Verification items for the finished model (mm, model axes). Round coordinates to 2 decimals unless told otherwise and drop trailing zeros. Write each loop counter-clockwise with the first axis right and the second up, starting at its lowest first coordinate (ties: lowest second). Pieces come first, ordered by that corner, then holes. Notation, with made-up numbers: M 34.25,73.25 L 82.25,73.25 A34 cw 82.25,111.25 Z; hole C 22,54.25 d4. An arc over 180 degrees is marked long. Write each question's results on one line, items separated by ' | '.
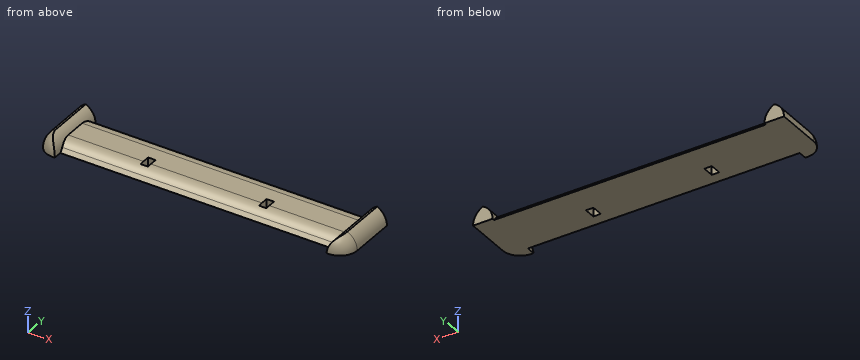
from build123d import *

# Parameters (mm, degrees)
F0_W          = 90
F0_H          = 18.32
F1_DEPTH      = 2.5
F2_W          = 2.16
F2_H          = 3.27
F3_DEPTH      = 25
F4_W          = 5
F4_H          = 18.32
F5_DEPTH      = 2.5
F6_T1_DEPTH   = 43.32
F6_T3_DEPTH   = 39.9706350946
F7_T1_DEPTH   = 39.9706350946
F7_T3_DEPTH   = 43.32
F8_T4_DEPTH   = 105.7168298797
F8_S5_R       = 5.0000000001
F8_T6_DEPTH   = 54
F8_S7_R       = 5.0000000001
F8_T8_DEPTH   = 54
F9_T4_DEPTH   = 105
F9_S5_R       = 5.0000000001
F9_T6_DEPTH   = 54
F9_S7_R       = 5.0000000001
F9_T8_DEPTH   = 54
F10_T4_ANGLE  = 350.8787991533
F10_S5_R      = 5.0000000001
F10_T6_DEPTH  = 9
F10_T10_ANGLE = 350.8787991654
F10_S11_R     = 5.0000000001
F10_T12_DEPTH = 9
F11_T4_DEPTH  = 90.3553390593
F11_S5_R      = 5.0000000001
F11_T6_DEPTH  = 47
F11_S7_R      = 5.0000000001
F11_T8_DEPTH  = 47


# Not quite as in the source:
# - a fillet or chamfer that OpenCascade refuses, or shapes differently, is made with other operations: its cross-section is extruded or revolved along the edge and cut away or added


with BuildPart() as f1:
    # F0 (on Top) → F1 (new body)
    with BuildSketch(Plane.XY):
        with Locations((28.5399998152, 34.3848172414)):
            Rectangle(F0_W, F0_H)
    extrude(amount=F1_DEPTH)

    # F2 (on face) → F3 (cut)
    with BuildSketch(Plane(origin=(0, 0, 0), x_dir=(1, 0, 0), z_dir=(0, 0, -1))):
        with Locations((11.4099998152, -32.7498172414)):
            Rectangle(F2_W, F2_H)
        with Locations((45.6699998152, -32.7498172414)):
            Rectangle(F2_W, F2_H)
    extrude(amount=-F3_DEPTH, mode=Mode.SUBTRACT)

    # F4 (on face) → F5 (join)
    with BuildSketch(Plane.XY.offset(2.5)):
        with Locations((-13.9600001848, 34.3848172414)):
            Rectangle(F4_W, F4_H)
        with Locations((71.0399998152, 34.3848172414)):
            Rectangle(F4_W, F4_H)
    extrude(amount=F5_DEPTH)

    # F6: fillet of radius 5 on 2 edges, made by hand

    # F6_s2 → F6_t1 (cut)
    with BuildSketch(Plane.XZ.offset(-56.0448172414)):
        with BuildLine():
            ThreePointArc((-16.4600001848, 0), (-14.9955340907, 3.5355339059), (-11.4600001848, 5))
            Line((-11.4600001848, 5), (-16.4600001848, 5))
            Line((-16.4600001848, 5), (-16.4600001848, 0))
        make_face()
    extrude(amount=F6_T1_DEPTH, mode=Mode.SUBTRACT)

    # F6_s4 → F6_t3 (cut)
    with BuildSketch(Plane.XZ.offset(-54.3701347887)):
        with BuildLine():
            ThreePointArc((-15.7901272037, 5), (-13.2901272037, 4.3301270189), (-11.4600001848, 2.5))
            Line((-11.4600001848, 2.5), (-11.4600001848, 5))
            Line((-11.4600001848, 5), (-15.7901272037, 5))
        make_face()
    extrude(amount=F6_T3_DEPTH, mode=Mode.SUBTRACT)

    # F7: fillet of radius 5 on 2 edges, made by hand

    # F7_s2 → F7_t1 (cut)
    with BuildSketch(Plane.XZ.offset(-54.3701347887)):
        with BuildLine():
            ThreePointArc((68.5399998152, 2.5), (70.3701268341, 4.3301270189), (72.8701268341, 5))
            Line((72.8701268341, 5), (68.5399998152, 5))
            Line((68.5399998152, 5), (68.5399998152, 2.5))
        make_face()
    extrude(amount=F7_T1_DEPTH, mode=Mode.SUBTRACT)

    # F7_s4 → F7_t3 (cut)
    with BuildSketch(Plane.XZ.offset(-56.0448172414)):
        with BuildLine():
            ThreePointArc((73.5399998152, 0), (72.0755337212, 3.5355339059), (68.5399998152, 5))
            Line((68.5399998152, 5), (73.5399998152, 5))
            Line((73.5399998152, 5), (73.5399998152, 0))
        make_face()
    extrude(amount=F7_T3_DEPTH, mode=Mode.SUBTRACT)

    # F8: chamfer of 5 on 1 edges, made by hand


with BuildPart() as f8_tool2:
    # F8_s3 → F8_t4 (new body)
    with BuildSketch(Plane.YZ.offset(-24.3184151246)):
        Polygon((30.2248172414, 2.5), (25.2248172414, -2.5), (25.2248172414, 2.5), align=None)
    extrude(amount=F8_T4_DEPTH)

    # F8_s5 → F8_t6 (cut, symmetric)
    with BuildSketch(Plane.XZ.offset(-27.7)):
        with Locations((-15.7901272038, -1e-10)):
            Circle(F8_S5_R)
    extrude(amount=F8_T6_DEPTH, both=True, mode=Mode.SUBTRACT)

    # F8_s7 → F8_t8 (cut, symmetric)
    with BuildSketch(Plane.XZ.offset(-27.7)):
        with Locations((72.8701268342, -1e-10)):
            Circle(F8_S7_R)
    extrude(amount=F8_T8_DEPTH, both=True, mode=Mode.SUBTRACT)


with BuildPart() as f1_1:
    add(f1.part)

    # F8_t1: cut F8_tool2
    add(f8_tool2.part, mode=Mode.SUBTRACT)

    # F9: fillet of radius 5 on 1 edges, made by hand


with BuildPart() as f9_tool2:
    # F9_s3 → F9_t4 (new body)
    with BuildSketch(Plane.YZ.offset(81.0399998152)):
        with BuildLine():
            ThreePointArc((43.5448172414, -2.5), (42.0803511473, 1.0355339059), (38.5448172414, 2.5))
            Line((38.5448172414, 2.5), (43.5448172414, 2.5))
            Line((43.5448172414, 2.5), (43.5448172414, -2.5))
        make_face()
    extrude(amount=-F9_T4_DEPTH)

    # F9_s5 → F9_t6 (cut, symmetric)
    with BuildSketch(Plane.XZ.offset(-41)):
        with Locations((72.8701268342, -1e-10)):
            Circle(F9_S5_R)
    extrude(amount=F9_T6_DEPTH, both=True, mode=Mode.SUBTRACT)

    # F9_s7 → F9_t8 (cut, symmetric)
    with BuildSketch(Plane.XZ.offset(-41)):
        with Locations((-15.7901272038, -1e-10)):
            Circle(F9_S7_R)
    extrude(amount=F9_T8_DEPTH, both=True, mode=Mode.SUBTRACT)


with BuildPart() as f1_2:
    add(f1_1.part)

    # F9_t1: cut F9_tool2
    add(f9_tool2.part, mode=Mode.SUBTRACT)

    # F10: fillet of radius 5 on 2 edges, made by hand


with BuildPart() as f10_tool2:
    # F10_s3 → F10_t4 (revolve)
    with BuildSketch(Plane(origin=(-4.0989769567, 0, -5.492965009), x_dir=(0, 1, 0), z_dir=(0.5980609221, 0, 0.8014506432))):
        with BuildLine():
            ThreePointArc((25.2248172414, 9.1846245187), (26.6892833355, 5.6490906128), (30.2248172414, 4.1846245187))
            Line((30.2248172414, 4.1846245187), (25.2248172414, 4.1846245187))
            Line((25.2248172414, 4.1846245187), (25.2248172414, 9.1846245187))
        make_face()
    revolve(axis=Axis((-11.4600001847, 25.2248172414, -1e-10), (0, 1, 0)), revolution_arc=F10_T4_ANGLE)

    # F10_s5 → F10_t6 (intersect, symmetric)
    with BuildSketch(Plane.XZ.offset(-27.7)):
        with Locations((-15.7901272038, -1e-10)):
            Circle(F10_S5_R)
    extrude(amount=F10_T6_DEPTH, both=True, mode=Mode.INTERSECT)


with BuildPart() as f1_3:
    add(f1_2.part)

    # F10_t1: cut F10_tool2
    add(f10_tool2.part, mode=Mode.SUBTRACT)


with BuildPart() as f10_tool8:
    # F10_s9 → F10_t10 (revolve)
    with BuildSketch(Plane(origin=(14.7214175546, 0, -28.147572216), x_dir=(0, 1, 0), z_dir=(0.4634498715, 0, -0.8861231385))):
        with BuildLine():
            ThreePointArc((25.2248172414, 60.7348797497), (26.6892833355, 57.1993458438), (30.2248172414, 55.7348797497))
            Line((30.2248172414, 55.7348797497), (25.2248172414, 55.7348797497))
            Line((25.2248172414, 55.7348797497), (25.2248172414, 60.7348797497))
        make_face()
    revolve(axis=Axis((68.5399998153, 25.2248172414, 1e-10), (0, 1, 0)), revolution_arc=F10_T10_ANGLE)

    # F10_s11 → F10_t12 (intersect, symmetric)
    with BuildSketch(Plane.XZ.offset(-27.7)):
        with Locations((72.8701268342, -1e-10)):
            Circle(F10_S11_R)
    extrude(amount=F10_T12_DEPTH, both=True, mode=Mode.INTERSECT)


with BuildPart() as f1_4:
    add(f1_3.part)

    # F10_t7: cut F10_tool8
    add(f10_tool8.part, mode=Mode.SUBTRACT)

    # F11: fillet of radius 5 on 1 edges, made by hand


with BuildPart() as f11_tool2:
    # F11_s3 → F11_t4 (new body)
    with BuildSketch(Plane.YZ.offset(-16.6376697145)):
        with BuildLine():
            ThreePointArc((28.7603511473, 1.0355339059), (30.3824678914, 2.1193976626), (32.2958850533, 2.5))
            Line((32.2958850533, 2.5), (30.2248172414, 2.5))
            Line((30.2248172414, 2.5), (28.7603511473, 1.0355339059))
        make_face()
    extrude(amount=F11_T4_DEPTH)

    # F11_s5 → F11_t6 (cut, symmetric)
    with BuildSketch(Plane.XZ.offset(-30.5)):
        with Locations((72.8701268342, -1e-10)):
            Circle(F11_S5_R)
    extrude(amount=F11_T6_DEPTH, both=True, mode=Mode.SUBTRACT)

    # F11_s7 → F11_t8 (cut, symmetric)
    with BuildSketch(Plane.XZ.offset(-30.5)):
        with Locations((-15.7901272038, -1e-10)):
            Circle(F11_S7_R)
    extrude(amount=F11_T8_DEPTH, both=True, mode=Mode.SUBTRACT)


with BuildPart() as f1_5:
    add(f1_4.part)

    # F11_t1: cut F11_tool2
    add(f11_tool2.part, mode=Mode.SUBTRACT)


solid = f1_5.part
1) Material ranges on line 1 (Z direction, x = -8, y = 35.75); line 2 (X direction, y = 32, z = 2.9); line 3 (X direction, y = 41.25, z = 3.3), recorded low to high. Write a range as [from, to].
Calculated:
line 1: z = [0, 2.5] | line 2: x = [-15.53, -11.72], [68.8, 72.61] | line 3: x = [-15.22, -12.03], [69.11, 72.3]
2) Depth check by flat-ended pin: P1, Ø1.1, axis at x = 11.5, z = 1, coming from the +Y side; P2, Ø0.6, axis at x = 12, z = 1.5, coming from the -Y side; P3, Ø1.7, axis at x = 46, z = 1.5, coming from the +Y side. Enter the tip coordinate at first touch or a pass-through.
Calculated:
P1: stops at y = 42.58 | P2: stops at y = 28.93 | P3: stops at y = 42.43
3) Sectioned sample at C-C, the plane x = 38.5. Record the cut outline in (y, z).
Calculated:
outline: M 27.72,0 L 42.87,0 A5 ccw 38.54,2.5 L 32.3,2.5 A5 ccw 28.76,1.04 Z
4) Sectioned sample at D-D, the plane y = 41.5. Record the cut outline in (x, z).
Calculated:
outline: M -16.46,0 L 73.54,0 A5 ccw 70.71,4.51 A5 ccw 68.11,1.53 L -11.03,1.53 A5 ccw -13.63,4.51 A5 ccw Z
5) Sectioned sample at A-A, the plane z = 3.2. Record the cut outline in (x, y), and give its area (3 significant figures).
Calculated:
outline: M -15.3,30.22 A3.84 ccw -11.95,26.41 L -11.95,43.54 L -15.3,43.54 Z; M 69.03,26.41 A3.84 ccw 72.38,30.22 L 72.38,43.54 L 69.03,43.54 Z | area: 109 mm²
6) Sectioned sample at B-B, the plane y = 36. Record the cut outline in (x, z).
Calculated:
outline: M -16.46,0 L 73.54,0 A5 ccw 70.71,4.51 A5 ccw 68.54,2.5 L -11.46,2.5 A5 ccw -13.63,4.51 A5 ccw Z
